Here's how the part is built. I have some questions about the finished solid (model axes, mm). A direction names the side the tool comes from. Round coordinates to 2 decimals unless told otherwise and drop trailing zeros. Loops run counter-clockwise (first coordinate to the right, second up) from the corner with the lowest first, then second, coordinate; pieces in that order, holes last. Notation, with made-up numbers: (12, -31) - (30, -31) arc R18 cw to (30, -20) - close; hole circle Ø2 at (0, 30). An arc over 180 degrees is marked (long way). Answer as a JSON object with one key per item and string values. Group by question number.
1) I want a section at B-B, the plane x = 59. Please give me the cut outline in (y, z).
2) Will these pins go through, and if not, where does the flat tip stop? P1, Ø5.5, axis at x = 140, z = 3, coming from the +Y side; P2, Ø2, axis at x = 165, z = 3, coming from the -Y side.
3) If we mould it in two halves opening along X, with no side actions, what happens to faces 3 (the face through (204.5, 0, 3)), 4 (the face through (115, -0.5, 5)), 5 (the face through (91.669, -2.226, 2.474)), 6 (the face through (101, -2, 9))? For each: pulls with the +X half, pulls with the -X half, needs draft (parallel to the pull), parting line crosses it, or undercut.
4) If I drill on line 1 along Z through (x, y) = (190, -2.35); line 2 along Y through (x, z) = (116.5, 4); line 3 along Z through (x, y) = (117.5, 1.5), over which ranges is the centre line in solid material (lowest first)? Write a range as [from, to].
5) Which directions (+Z, -Z, +X, -X, +Y, -Y) give clear straight access to the entire face, cutting with the end or side of a thin tool? Please do faces 1 (the face through (116.669, -2.226, 2.474)), 2 (the face through (42, -0.5, 3)).
from build123d import *

# Parameters (mm, degrees)
BOSS_EXTRUDE1_DEPTH = 480
SKETCH2_R           = 1.75
CUT_EXTRUDE1_DEPTH  = 60
SKETCH3_R           = 3
CUT_EXTRUDE2_DEPTH  = 4.5
SKETCH4_R           = 0.5
CUT_EXTRUDE3_DEPTH  = 14.5
LPATTERN1_COUNT     = 19
LPATTERN1_PITCH     = 25
SKETCH5_W           = 307.473563077
SKETCH5_H           = 32.361597021
CUT_EXTRUDE4_DEPTH  = 9


with BuildPart() as part:
    # Sketch1 → Boss-Extrude1 (new body)
    with BuildSketch(Plane(origin=(0, 0, 0), x_dir=(0, 0, -1), z_dir=(1, 0, 0))):
        with BuildLine():
            Line((-3, -4), (2.6, -4))
            Line((2.6, -4), (3, -3.6))
            Line((3, -3.6), (3, 0.64))
            ThreePointArc((3, 0.64), (2.717157288, 0.757157288), (2.6, 1.04))
            Line((2.6, 1.04), (2.5, 1.15))
            Line((2.5, 1.15), (2.2, 1.15))
            ThreePointArc((2.2, 1.15), (1.75, 1.6), (2.2, 2.05))
            Line((2.2, 2.05), (2.5, 2.05))
            Line((2.5, 2.05), (2.6, 2.16))
            ThreePointArc((2.6, 2.16), (2.717157288, 2.442842712), (3, 2.56))
            Line((3, 2.56), (3, 3.6))
            Line((3, 3.6), (2.6, 4))
            Line((2.6, 4), (-3, 4))
            Line((-3, 4), (-3, -4))
        make_face()
    boss_extrude1 = extrude(amount=BOSS_EXTRUDE1_DEPTH)

    # Mirror1: Boss-Extrude1 across plane
    add(boss_extrude1.mirror(Plane(origin=(480, -4, 3), x_dir=(1, 0, 0), z_dir=(0, 0, -1))))

    # Sketch2 → Cut-Extrude1 (cut)
    with BuildSketch(Plane(origin=(0, 4, 0), x_dir=(1, 0, 0), z_dir=(0, 1, 0))):
        with Locations((15, -3)):
            Circle(SKETCH2_R)
    cut_extrude1 = extrude(amount=-CUT_EXTRUDE1_DEPTH, mode=Mode.SUBTRACT)

    # Sketch3 → Cut-Extrude2 (cut)
    with BuildSketch(Plane(origin=(0, 4, 0), x_dir=(1, 0, 0), z_dir=(0, 1, 0))):
        with Locations((15, -3)):
            Circle(SKETCH3_R)
    cut_extrude2 = extrude(amount=-CUT_EXTRUDE2_DEPTH, mode=Mode.SUBTRACT)

    # Sketch4 → Cut-Extrude3 (cut)
    with BuildSketch(Plane(origin=(0, 4, 0), x_dir=(1, 0, 0), z_dir=(0, 1, 0))):
        with Locations((0, -3)):
            Circle(SKETCH4_R)
    extrude(amount=-CUT_EXTRUDE3_DEPTH, mode=Mode.SUBTRACT)

    # LPattern1: Cut-Extrude1, Cut-Extrude2 ×19
    with Locations(*[(i * LPATTERN1_PITCH, 0, 0) for i in range(1, LPATTERN1_COUNT)]):
        add(cut_extrude1, mode=Mode.SUBTRACT)
        add(cut_extrude2, mode=Mode.SUBTRACT)

    # Sketch5 → Cut-Extrude4 (cut, through all)
    with BuildSketch(Plane.XZ.offset(4)):
        with Locations((358.236781539, 13.180798511)):
            Rectangle(SKETCH5_W, SKETCH5_H)
    extrude(amount=-CUT_EXTRUDE4_DEPTH, mode=Mode.SUBTRACT)


solid = part.part
Outcome:
{
 "1": {"outline": "(-4, -2.6) - (-3.6, -3) - (0.64, -3) arc R0.4 cw to (1.04, -2.6) - (1.15, -2.5) - (1.15, -2.2) arc R0.45 cw to (2.05, -2.2) - (2.05, -2.5) - (2.16, -2.6) arc R0.4 cw to (2.56, -3) - (3.6, -3) - (4, -2.6) - (4, 8.6) - (3.6, 9) - (2.56, 9) arc R0.4 cw to (2.16, 8.6) - (2.05, 8.5) - (2.05, 8.2) arc R0.45 cw to (1.15, 8.2) - (1.15, 8.5) - (1.04, 8.6) arc R0.4 cw to (0.64, 9) - (-3.6, 9) - (-4, 8.6) - close"},
 "2": {"P1": "y = -0.5", "P2": "through"},
 "3": {"face 3": "pulls with the +X half", "face 4": "undercut", "face 5": "undercut", "face 6": "needs draft"},
 "4": {"line 1": "[-3, 1.25], [4.75, 9]", "line 2": "[-4, -0.5]", "line 3": "[-1.76, 1.34], [4.66, 7.76]"},
 "5": {"face 1": "+Y, -Y", "face 2": "+Y"}
}
